```python
from build123d import *

# Parameters (mm, degrees)
ESQUISSE1_W             = 40
ESQUISSE1_H             = 40
ESQUISSE1_R             = 16
BOSS_EXTRU_1_DEPTH      = 30
ESQUISSE2_W             = 40
ESQUISSE2_H             = 40
BOSS_EXTRU_2_DEPTH      = 5
ESQUISSE3_R             = 1.5
ENL_V_MAT_EXTRU_1_DEPTH = 5
ESQUISSE4_R             = 10
ENL_V_MAT_EXTRU_2_DEPTH = 5
ESQUISSE5_R             = 10
BOSS_EXTRU_3_DEPTH      = 10
ESQUISSE6_R             = 12
BOSS_EXTRU_4_DEPTH      = 1
ESQUISSE7_R             = 8.5
BOSS_EXTRU_5_DEPTH      = 14.25
ESQUISSE8_R             = 12
BOSS_EXTRU_6_DEPTH      = 1
ESQUISSE9_W             = 40
ESQUISSE9_H             = 40
ESQUISSE9_R             = 2.75
ESQUISSE9_R_2           = 10
BOSS_EXTRU_7_DEPTH      = 4
ESQUISSE10_R            = 1.5
ESQUISSE10_R_2          = 2
ENL_V_MAT_EXTRU_3_DEPTH = 65.25
CHANFREIN1_SIZE         = 4


with BuildPart() as part:
    # Esquisse1 → Boss.-Extru.1 (new body)
    with BuildSketch(Plane.XY):
        Rectangle(ESQUISSE1_W, ESQUISSE1_H)
        Circle(ESQUISSE1_R, mode=Mode.SUBTRACT)
    extrude(amount=BOSS_EXTRU_1_DEPTH)

    # Esquisse2 → Boss.-Extru.2 (add)
    with BuildSketch(Plane.XY.offset(30)):
        Rectangle(ESQUISSE2_W, ESQUISSE2_H)
    extrude(amount=BOSS_EXTRU_2_DEPTH)

    # Esquisse3 → Enl_v. mat.-Extru.1 (cut)
    with BuildSketch(Plane.XY.offset(35)):
        with Locations((0, 13)):
            Circle(ESQUISSE3_R)
        with Locations((13, 0)):
            Circle(ESQUISSE3_R)
        with Locations((0, -13)):
            Circle(ESQUISSE3_R)
        with Locations((-13, 0)):
            Circle(ESQUISSE3_R)
    extrude(amount=-ENL_V_MAT_EXTRU_1_DEPTH, mode=Mode.SUBTRACT)

    # Esquisse4 → Enl_v. mat.-Extru.2 (cut)
    with BuildSketch(Plane.XY.offset(35)):
        Circle(ESQUISSE4_R)
    extrude(amount=-ENL_V_MAT_EXTRU_2_DEPTH, mode=Mode.SUBTRACT)

    # Esquisse5 → Boss.-Extru.3 (add)
    with BuildSketch(Plane.ZY.offset(20)):
        with Locations((21, 0)):
            Circle(ESQUISSE5_R)
    extrude(amount=BOSS_EXTRU_3_DEPTH)

    # Esquisse6 → Boss.-Extru.4 (add)
    with BuildSketch(Plane.ZY.offset(20)):
        with Locations((21, 0)):
            Circle(ESQUISSE6_R)
    extrude(amount=BOSS_EXTRU_4_DEPTH)

    # Esquisse7 → Boss.-Extru.5 (add)
    with BuildSketch(Plane(origin=(20, 0, 0), x_dir=(0, 0, -1), z_dir=(1, 0, 0))):
        with Locations((-21, 0)):
            Circle(ESQUISSE7_R)
    extrude(amount=BOSS_EXTRU_5_DEPTH)

    # Esquisse8 → Boss.-Extru.6 (add)
    with BuildSketch(Plane(origin=(20, 0, 0), x_dir=(0, 0, -1), z_dir=(1, 0, 0))):
        with Locations((-21, 0)):
            Circle(ESQUISSE8_R)
    extrude(amount=BOSS_EXTRU_6_DEPTH)

    # Esquisse9 → Boss.-Extru.7 (add)
    with BuildSketch(Plane.XY.offset(35)):
        Rectangle(ESQUISSE9_W, ESQUISSE9_H)
        with Locations((0, 13)):
            Circle(ESQUISSE9_R, mode=Mode.SUBTRACT)
        with Locations((-13, 0)):
            Circle(ESQUISSE9_R, mode=Mode.SUBTRACT)
        with Locations((0, -13)):
            Circle(ESQUISSE9_R, mode=Mode.SUBTRACT)
        with Locations((13, 0)):
            Circle(ESQUISSE9_R, mode=Mode.SUBTRACT)
        Circle(ESQUISSE9_R_2, mode=Mode.SUBTRACT)
    extrude(amount=BOSS_EXTRU_7_DEPTH)

    # Esquisse10 → Enl_v. mat.-Extru.3 (cut, through all)
    with BuildSketch(Plane(origin=(34.25, 0, 0), x_dir=(0, 0, -1), z_dir=(1, 0, 0))):
        with Locations((-21, 6)):
            Circle(ESQUISSE10_R)
        with Locations((-15.803847577, -3)):
            Circle(ESQUISSE10_R)
        with Locations((-26.196152423, -3)):
            Circle(ESQUISSE10_R)
        with Locations((-21, 0)):
            Circle(ESQUISSE10_R_2)
    extrude(amount=-ENL_V_MAT_EXTRU_3_DEPTH, mode=Mode.SUBTRACT)

    # Chanfrein1
    chanfrein1_edges = [part.edges().sort_by_distance(p)[0] for p in [
        (-20, 20, 19.5),
        (20, 20, 19.5),
        (20, -20, 19.5),
        (-20, -20, 19.5),
    ]]
    chamfer(chanfrein1_edges, length=CHANFREIN1_SIZE)


solid = part.part
```
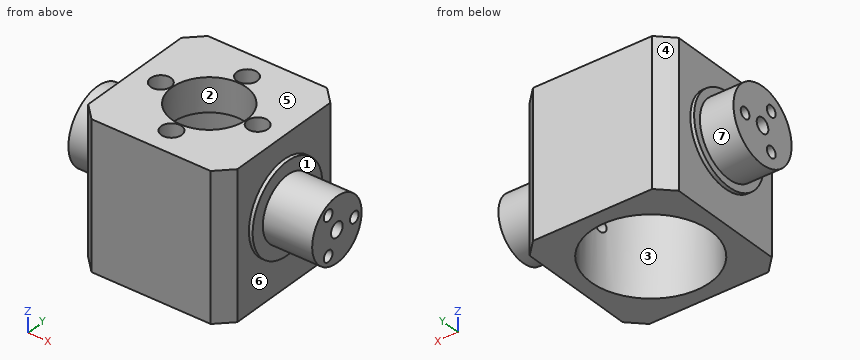
CAD build for the part. Positions are in the model's coordinates, mm. Face numbers are marked on the shaded views. A direction names the side the tool comes from. Round coordinates to 2 decimals unless told otherwise and drop trailing zeros. Write each loop counter-clockwise with the first axis right and the second up, starting at its lowest first coordinate (ties: lowest second). Pieces come first, ordered by that corner, then holes. Notation, with made-up numbers: (54, -33.75) - (97, -33.75) arc R24 ccw to (97, 2.25) - close; hole circle Ø10 at (39.25, -35.5). An arc over 180 degrees is marked (long way). Write item = value, one per line. Start each with the question number.
Q1. Which spindle directions (+Z, -Z, +X, -X, +Y, -Y) get a long thin tool onto all of the face, cutting with end or side? Do the marked faces 5, 6 and 7. Say none if no direction does.
Q2. Mould opens along X. For the marked faces 1, 2, 3 and 4 say: pulls with the +X half, pulls with the -X half, needs draft (parallel to the pull), parting line crosses it, or undercut.
Q3. Band-saw the part on B-B (z = 7). Give the cut face in (x, y), then the cut area to 3 significant figures.
Q4. Band-saw the part on C-C (y = 13). Give the cut face in (x, z), then the cut area to 3 significant figures.
Q5. Band-saw the part on A-A (x = 25.5). Give the cut face in (y, z), then the cut area to 3 significant figures.
Q6. Probe L1, parallel to Y at x = -25.5, z = 21; L2, parallel to Y at x = 0, z = 36.25; L3, parallel to Y at x = 0, z = 34.5. List the from-to ranges inside material, lowest first. Write a range as from..to.
Q7. Drop flat-ended pins along their axis: pin 1 (3.5 mm diameter, centred on x = 0, y = -13, fed in from -Z); pin 2 (8 mm diameter, centred on x = 26, z = 7, fed in from +Y); pin 3 (3 mm diameter, centred on x = 0.5, y = -13.5, fed in from +Z); pin 4 (4 mm diameter, centred on y = -9, z = 6.5, fed in from +X). Give the stop position or say it passes through.
Answers below:
q1.face_5 = +Z, +X, -X, +Y, -Y
q1.face_6 = +X
q1.face_7 = -X
q2.face_1 = pulls with the +X half
q2.face_2 = undercut
q2.face_3 = undercut
q2.face_4 = pulls with the -X half
q3.outline = (-20, -16) - (-16, -20) - (16, -20) - (20, -16) - (20, 16) - (16, 20) - (-16, 20) - (-20, 16) - close; hole circle Ø32 at (0, 0)
q3.area = 764 mm2
q4.outline = (-20, 0) - (-9.33, 0) - (-9.33, 30) - (-1.5, 30) - (-1.5, 35) - (-2.75, 35) - (-2.75, 39) - (-20, 39) - close; (1.5, 30) - (9.33, 30) - (9.33, 0) - (20, 0) - (20, 39) - (2.75, 39) - (2.75, 35) - (1.5, 35) - close
q4.area = 963 mm2
q5.outline = circle Ø17 at (0, 21); hole circle Ø3 at (-3, 15.8); hole circle Ø3 at (-3, 26.2); hole circle Ø4 at (0, 21); hole circle Ø3 at (6, 21)
q5.area = 193 mm2
q6.L1 = -10..-2, 2..4.5, 7.5..10
q6.L2 = -20..-15.75, -10.25..-10, 10..10.25, 15.75..20
q6.L3 = -20..-14.5, -11.5..-10, 10..11.5, 14.5..20
q7.pin_1 = 30
q7.pin_2 = through
q7.pin_3 = 35
q7.pin_4 = 20
